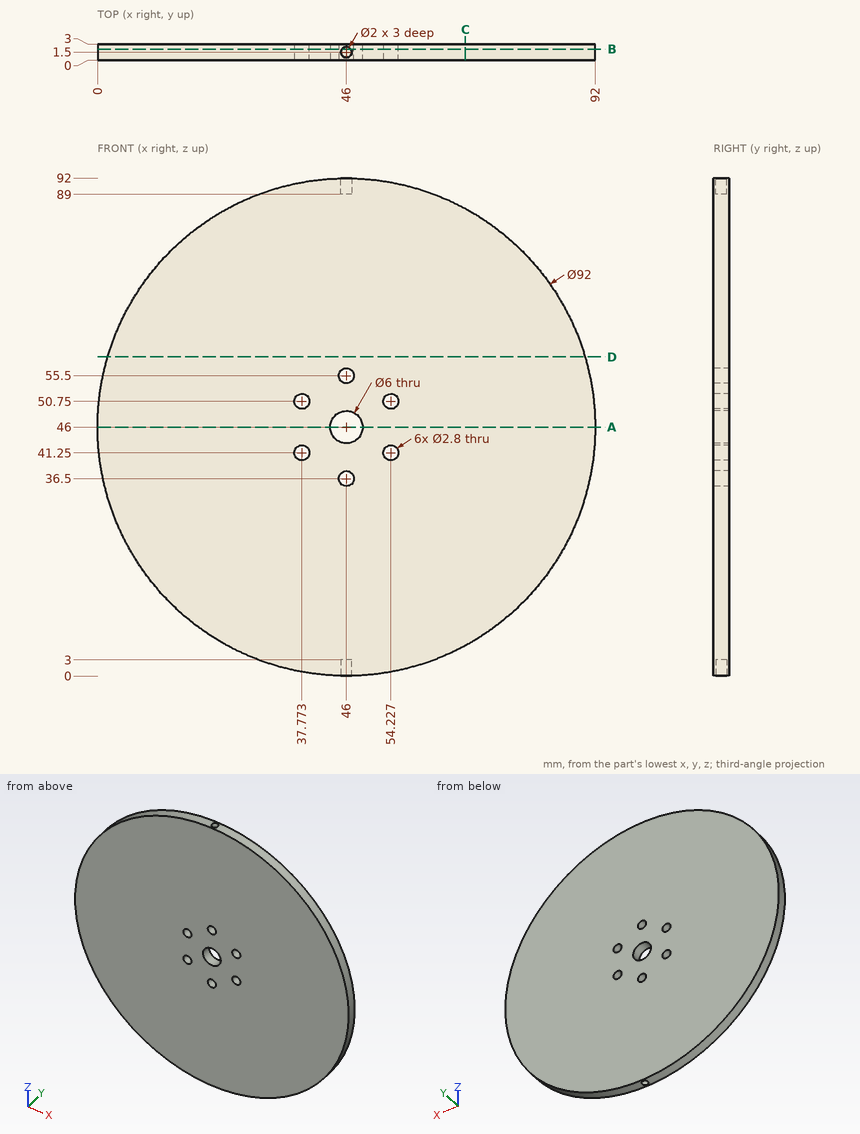
Here's the drawing with two shaded views (mm, measured from the low corner). I have some questions. Round coordinates to 2 decimals unless told otherwise and drop trailing zeros. Loops run counter-clockwise (first coordinate to the right, second up) from the corner with the lowest first, then second, coordinate; pieces in that order, holes last. Notation, with made-up numbers: M 25.25,43 L 71.25,43 A25 ccw 71.25,67 Z; hole C 25.5,42.25 d10. An arc over 180 degrees is marked long. Answer as a JSON object with one key per item and string values. Group by question number.
Q1. Imagine slicing it at C-C, the plane x = 68. Please give me the cut outline in (y, z), then the cut area to 3 significant figures.
Q2. Please list where these lines run through material, in increasing order: L1, parallel to Z at x = 46, y = 1.7; L2, parallel to Y at x = 46, z = 1.4; L3, parallel to Z at x = 45, y = 0.8.
Q3. Imagine slicing it at B-B, the plane y = 2.05. Count the separate pieces of the cut face and the enclosed holes in it, then the cut area to 3 significant figures.
Q4. Imagine slicing it at D-D, the plane z = 59. Please give me the cut outline in (x, y) (1 decimal), then the cut area to 3 significant figures.
Q5. Will these pins go through, and if not, where does the flat tip stop? pin 1 (0.6 mm diameter, centred on x = 45.5, y = 1.5, fed in from +Z); pin 2 (1.7 mm diameter, centred on x = 46, z = 36.5, fed in from -Y); pin 3 (1.8 mm diameter, centred on x = 46, y = 1.5, fed in from -Z); pin 4 (1 mm diameter, centred on x = 64, y = 1.5, fed in from +Z).
Q6. Imagine slicing it at A-A, the plane z = 46. Please give me the cut outline in (x, y), then the cut area to 3 significant figures.
Findings:
{
 "1": {"outline": "M 0,5.6 L 3,5.6 L 3,86.4 L 0,86.4 Z", "area": "242 mm2"},
 "2": {"L1": "z = 3 to 35.1, 37.9 to 43, 49 to 54.1, 56.9 to 89", "L2": "y = 0 to 0.5, 2.5 to 3", "L3": "z = 0.01 to 35.52, 37.48 to 43.17, 48.83 to 54.52, 56.48 to 91.99"},
 "3": {"separate pieces": "1", "enclosed holes": "7", "area": "6,570 mm2"},
 "4": {"outline": "M 1.9,0 L 90.1,0 L 90.1,3 L 1.9,3 Z", "area": "265 mm2"},
 "5": {"pin 1": "stops at z = 89", "pin 2": "passes through", "pin 3": "stops at z = 3", "pin 4": "stops at z = 88.54"},
 "6": {"outline": "M 0,0 L 43,0 L 43,3 L 0,3 Z; M 49,0 L 92,0 L 92,3 L 49,3 Z", "area": "258 mm2"}
}
